Could you check a few things on this model? Use its own coordinates, in mm. Face numbers are marked on the shaded views. A direction names the side the tool comes from. Round coordinates to 2 decimals unless told otherwise and drop trailing zeros. Loops run counter-clockwise (first coordinate to the right, second up) from the corner with the lowest first, then second, coordinate; pieces in that order, holes last. Notation, with made-up numbers: (65, -36.75) -> (115, -36.75) arc R9 cw to (115, -21.75) -> close; hole circle Ø9 at (26, -17.75). An arc over 180 degrees is marked (long way). Put each result on its own line as item: value. Start each with the question number.
1. Imagine slicing it at D-D, the plane x = 0. Please give me the cut outline in (y, z) (3 decimals), and give its area (3 significant figures).
2. Which directions (+Z, -Z, +X, -X, +Y, -Y) give clear straight access to the entire face, cutting with the end or side of a thin tool? Please do the marked faces 5, 6 and 7.
3. If we mould it in two halves opening along Z, with no side actions, what happens to the marked faces 1, 2, 3 and 4? For each: pulls with the +Z half, pulls with the -Z half, needs draft (parallel to the pull), parting line crosses it, or undercut.
4. Imagine slicing it at B-B, the plane y = -5. Please give me the cut outline in (x, z).
5. I need wall thicknesses on line 1 (X direction, y = 5, z = -13); line 2 (X direction, y = -4, z = -4); line 3 (Z direction, x = -19, y = -4). Which ranges of each line are inside material? Lowest first, please. Write a range as [from, to].
6. Imagine slicing it at A-A, the plane y = 4. Please give me the cut outline in (x, z), and give its area (3 significant figures).
7. I'm going to push flat-ended pins straight in: P1, Ø2.5, axis at x = 2.5, z = 16.5, coming from the +Y side (3 decimals); P2, Ø9.5, axis at x = -19.05, z = -12.7, coming from the +Y side (3 decimals). Where does each tip first touch, or does it pass through?
```python
from build123d import *

# Parameters (mm, degrees)
EXTRUDE1_DEPTH          = 19.05
CUT_EXTRUDE1_DEPTH      = 51.8
FILLET1_R               = 3.175
CUT_EXTRUDE2_DEPTH      = 2.54
CUT_EXTRUDE2_DEPTH_BACK = 7.35
SKETCH4_R               = 3.5687
CUT_EXTRUDE3_DEPTH      = 32.7500001


with BuildPart() as part:
    # Sketch1 → Extrude1 (new body, symmetric)
    with BuildSketch(Plane.XY):
        Polygon((25.4, 15.875), (12.827, 15.875), (12.827, -9.525), (-12.827, -9.525), (-12.827, 15.875), (-25.4, 15.875), (-25.4, -15.875), (25.4, -15.875), align=None)
    extrude(amount=EXTRUDE1_DEPTH, both=True)

    # Sketch2 → Cut-Extrude1 (cut, through all)
    with BuildSketch(Plane.ZY.offset(25.4)):
        with BuildLine():
            Line((-6.3627, 15.875), (-6.3627, 3.175))
            ThreePointArc((-6.3627, 3.175), (0, -3.1877), (6.3627, 3.175))
            Line((6.3627, 3.175), (6.3627, 15.875))
            Line((6.3627, 15.875), (-6.3627, 15.875))
        make_face()
    extrude(amount=-CUT_EXTRUDE1_DEPTH, mode=Mode.SUBTRACT)

    # Fillet1
    fillet1_edges = [part.edges().sort_by_distance(p)[0] for p in [
        (-12.827, -9.525, 0),
        (12.827, -9.525, 0),
    ]]
    fillet(fillet1_edges, radius=FILLET1_R)

    # Sketch3 → Cut-Extrude2 (cut, two sides)
    with BuildSketch(Plane(origin=(0, -9.525, 0), x_dir=(-1, 0, 0), z_dir=(0, 1, 0))) as cut_extrude2_sk:
        with BuildLine():
            Line((-11.1125, 4.7752), (-11.1125, -4.7752))
            ThreePointArc((-11.1125, -4.7752), (0, -15.8877), (11.1125, -4.7752))
            Line((11.1125, -4.7752), (11.1125, 4.7752))
            ThreePointArc((11.1125, 4.7752), (0, 15.8877), (-11.1125, 4.7752))
        make_face()
    extrude(amount=CUT_EXTRUDE2_DEPTH, mode=Mode.SUBTRACT)
    extrude(cut_extrude2_sk.sketch, amount=-CUT_EXTRUDE2_DEPTH_BACK, mode=Mode.SUBTRACT)

    # Sketch4 → Cut-Extrude3 (cut, through all)
    with BuildSketch(Plane(origin=(0, 15.875, 0), x_dir=(-1, 0, 0), z_dir=(0, 1, 0))):
        with Locations(Location((-19.05, -12.7, 0), (0, 0, 90))):  # turned: the seam where the file's is
            Circle(SKETCH4_R)
        with Locations(Location((-19.05, 12.7, 0), (0, 0, 90))):  # turned: the seam where the file's is
            Circle(SKETCH4_R)
        with Locations(Location((19.05, 12.7, 0), (0, 0, 90))):  # turned: the seam where the file's is
            Circle(SKETCH4_R)
        with Locations(Location((19.05, -12.7, 0), (0, 0, 90))):  # turned: the seam where the file's is
            Circle(SKETCH4_R)
    extrude(amount=-CUT_EXTRUDE3_DEPTH, mode=Mode.SUBTRACT)


solid = part.part
```
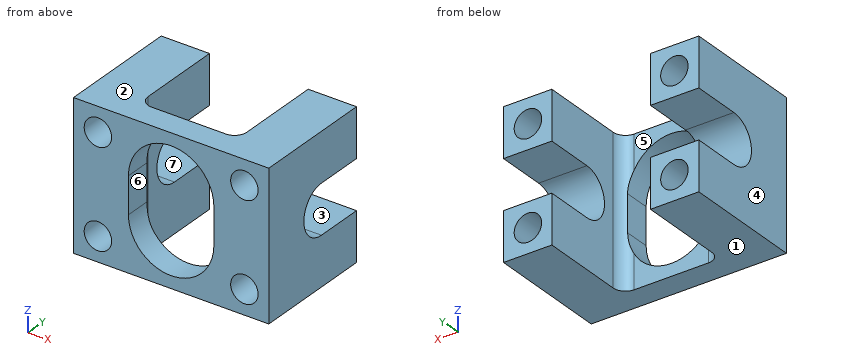
Entries:
1. outline: (-15.875, -19.05) -> (-9.525, -19.05) -> (-9.525, -15.888) -> (-15.875, -15.888) -> close; (-15.875, 15.888) -> (-9.525, 15.888) -> (-9.525, 19.05) -> (-15.875, 19.05) -> close
1. area: 40.2 mm^2
2. face 5: +Z, -Z, +Y
2. face 6: +Y, -Y
2. face 7: +X, -X, +Y
3. face 1: pulls with the -Z half
3. face 2: pulls with the +Z half
3. face 3: undercut
3. face 4: needs draft
4. outline: (-25.4, -19.05) -> (-12.83, -19.05) -> (-12.83, 19.05) -> (-25.4, 19.05) -> close; (12.83, -19.05) -> (25.4, -19.05) -> (25.4, 19.05) -> (12.83, 19.05) -> close; hole circle Ø7.14 at (-19.05, -12.7); hole circle Ø7.14 at (-19.05, 12.7); hole circle Ø7.14 at (19.05, -12.7); hole circle Ø7.14 at (19.05, 12.7)
5. line 1: [-25.4, -22.61], [-15.49, -12.83], [12.83, 15.49], [22.61, 25.4]
5. line 2: [-25.4, -12.83], [12.83, 25.4]
5. line 3: [-19.05, -16.27], [-9.13, 9.13], [16.27, 19.05]
6. outline: (-25.4, -19.05) -> (-12.83, -19.05) -> (-12.83, -6.36) -> (-25.4, -6.36) -> close; (-25.4, 6.36) -> (-12.83, 6.36) -> (-12.83, 19.05) -> (-25.4, 19.05) -> close; (12.83, -19.05) -> (25.4, -19.05) -> (25.4, -6.36) -> (12.83, -6.36) -> close; (12.83, 6.36) -> (25.4, 6.36) -> (25.4, 19.05) -> (12.83, 19.05) -> close; hole circle Ø7.14 at (-19.05, -12.7); hole circle Ø7.14 at (-19.05, 12.7); hole circle Ø7.14 at (19.05, -12.7); hole circle Ø7.14 at (19.05, 12.7)
6. area: 478 mm^2
7. P1: y = -9.525
7. P2: y = 15.875
